```python
from build123d import *

# Parameters (mm, degrees)
SKIZZE1_W                       = 42
SKIZZE1_H                       = 42
AUFSATZ_LINEAR_AUSTRAGEN1_DEPTH = 42
VERRUNDUNG1_R                   = 1
SKIZZE2_W                       = 40.5
SKIZZE2_H                       = 40.5
SCHNITT_LINEAR_AUSTRAGEN1_DEPTH = 1


with BuildPart() as part:
    # Skizze1 → Aufsatz-Linear austragen1 (new body)
    with BuildSketch(Plane(origin=(0, 0, 0), x_dir=(1, 0, 0), z_dir=(0, 1, 0))):
        with Locations((21, 21)):
            Rectangle(SKIZZE1_W, SKIZZE1_H)
    extrude(amount=AUFSATZ_LINEAR_AUSTRAGEN1_DEPTH)

    # Verrundung1
    verrundung1_edges = [part.edges().sort_by_distance(p)[0] for p in [
        (42, 21, 0),
        (0, 21, 0),
        (0, 21, -42),
        (42, 21, -42),
    ]]
    fillet(verrundung1_edges, radius=VERRUNDUNG1_R)

    # Skizze2 → Schnitt-Linear austragen1 (cut)
    with BuildSketch(Plane(origin=(0, 0, 0), x_dir=(1, 0, 0), z_dir=(0, 1, 0))):
        with Locations((21, 21)):
            Rectangle(SKIZZE2_W, SKIZZE2_H)
    extrude(amount=SCHNITT_LINEAR_AUSTRAGEN1_DEPTH, mode=Mode.SUBTRACT)


solid = part.part
```
Model file for the job. Use its own axes, mm. Round coordinates to 2 decimals unless told otherwise and drop trailing zeros. Order: outer loops, then holes, each group sorted by start corner. A loop starts at its lowest first (then second) coordinate and runs counter-clockwise, first axis right, second up. Notation, with made-up numbers: M 81.25,4 L 129.25,4 A19 cw 129.25,32 Z; hole C 14.5,66.5 d5. An arc over 180 degrees is marked long. Use CSV: the item, a comma, the result in double quotes.
Item 1: Probe probe 1 along Y at (x, z) = (31, -10). List the from-to ranges inside material, lowest first.
Worked answers:
probe 1,"1 to 42"
Item 2: Pull direction Z, two halves, no side cores. Call faces 1 (the face through (21, 21, 0)), 2 (the face through (0, 21, -21)), 3 (the face through (21, 1, -21)): released by +Z, released by -Z, zero draft, split by the parting line, or undercut.
Worked answers:
face 1,"released by +Z"
face 2,"zero draft"
face 3,"undercut"
Item 3: Saw through at A-A (z = -18). List the corners of the cut face in (x, y).
Worked answers:
outline,"M 0,0 L 0.75,0 L 0.75,1 L 41.25,1 L 41.25,0 L 42,0 L 42,42 L 0,42 Z"
Item 4: Saw through at B-B (x = 24.5). List the corners of the cut face in (y, z).
Worked answers:
outline,"M 0,-42 L 42,-42 L 42,0 L 0,0 L 0,-0.75 L 1,-0.75 L 1,-41.25 L 0,-41.25 Z"
